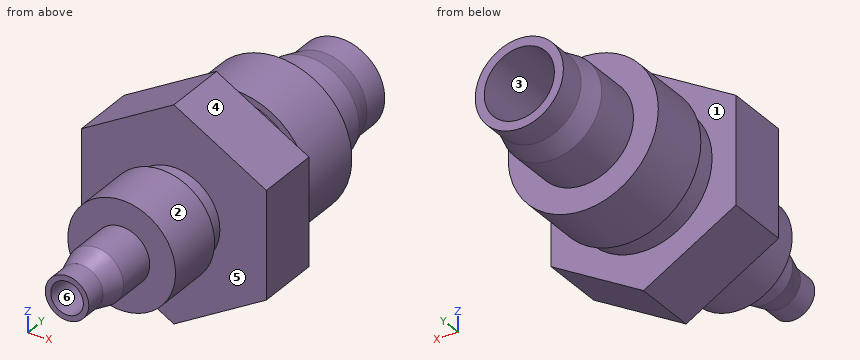
```python
from build123d import *

# Parameters (mm, degrees)
F1_DEPTH  = 3
F2_R      = 6.3
F3_DEPTH  = 2.5
F4_R      = 6.9
F5_DEPTH  = 6
F6_R      = 4.625
F7_DEPTH  = 4.5
F8_R      = 4.625
F9_DEPTH  = 2
F9_TAPER  = 16
F10_R     = 4.0515092285
F10_R_2   = 4
F11_DEPTH = 2.5
F12_R     = 3.225
F13_DEPTH = 20.5
F14_R     = 4.225
F15_DEPTH = 1.85
F16_R     = 4.95
F17_DEPTH = 5.5
F18_R     = 2.575
F19_DEPTH = 3.7
F20_R     = 2.575
F21_DEPTH = 2
F21_TAPER = 16
F22_R     = 2
F23_DEPTH = 2
F24_R     = 1.5
F25_DEPTH = 18.05
F26_R     = 3.225
F27_DEPTH = 3.5
F27_TAPER = 35


with BuildPart() as f1:
    # F0 (on Front) → F1 (new body, symmetric)
    with BuildSketch(Plane.XZ):
        Polygon((-8.5, -4.9074772881), (0, -9.8149545762), (8.5, -4.9074772881), (8.5, 4.9074772881), (0, 9.8149545762), (-8.5, 4.9074772881), align=None)
    extrude(amount=F1_DEPTH, both=True)

    # F2 (on face) → F3 (join)
    with BuildSketch(Plane(origin=(0, 3, 0), x_dir=(-1, 0, 0), z_dir=(0, 1, 0))):
        Circle(F2_R)
    extrude(amount=F3_DEPTH)

    # F4 (on face) → F5 (join)
    with BuildSketch(Plane(origin=(0, 5.5, 0), x_dir=(-1, 0, 0), z_dir=(0, 1, 0))):
        Circle(F4_R)
    extrude(amount=F5_DEPTH)

    # F6 (on face) → F7 (join)
    with BuildSketch(Plane(origin=(0, 11.5, 0), x_dir=(-1, 0, 0), z_dir=(0, 1, 0))):
        Circle(F6_R)
    extrude(amount=F7_DEPTH)

    # F8 (on face) → F9 (join)
    with BuildSketch(Plane(origin=(0, 16, 0), x_dir=(-1, 0, 0), z_dir=(0, 1, 0))):
        Circle(F8_R)
    extrude(amount=F9_DEPTH, taper=F9_TAPER)

    # F10 (on face) → F11 (join)
    with BuildSketch(Plane(origin=(0, 18, 0), x_dir=(-1, 0, 0), z_dir=(0, 1, 0))):
        Circle(F10_R)
        Circle(F10_R_2, mode=Mode.SUBTRACT)
        Circle(F10_R_2)
    extrude(amount=F11_DEPTH)

    # F12 (on face) → F13 (cut, through all)
    with BuildSketch(Plane(origin=(0, 20.5, 0), x_dir=(-1, 0, 0), z_dir=(0, 1, 0))):
        Circle(F12_R)
    extrude(amount=-F13_DEPTH, mode=Mode.SUBTRACT)

    # F14 (on face) → F15 (join)
    with BuildSketch(Plane.XZ.offset(3)):
        Circle(F14_R)
    extrude(amount=F15_DEPTH)

    # F16 (on face) → F17 (join)
    with BuildSketch(Plane.XZ.offset(4.85)):
        Circle(F16_R)
    extrude(amount=F17_DEPTH)

    # F18 (on face) → F19 (join)
    with BuildSketch(Plane.XZ.offset(10.35)):
        Circle(F18_R)
    extrude(amount=F19_DEPTH)

    # F20 (on face) → F21 (join)
    with BuildSketch(Plane.XZ.offset(14.05)):
        Circle(F20_R)
    extrude(amount=F21_DEPTH, taper=F21_TAPER)

    # F22 (on face) → F23 (join)
    with BuildSketch(Plane.XZ.offset(16.05)):
        Circle(F22_R)
    extrude(amount=F23_DEPTH)

    # F24 (on face) → F25 (cut, through all)
    with BuildSketch(Plane.XZ.offset(18.05)):
        Circle(F24_R)
    extrude(amount=-F25_DEPTH, mode=Mode.SUBTRACT)

    # F26 (on Front) → F27 (cut)
    with BuildSketch(Plane.XZ):
        Circle(F26_R)
    extrude(amount=F27_DEPTH, taper=F27_TAPER, mode=Mode.SUBTRACT)


solid = f1.part
```
Work out the finished part from the listing and answer in its coordinate system (mm). Face numbers are marked on the shaded views. A direction names the side the tool comes from. Round coordinates to 2 decimals unless told otherwise and drop trailing zeros. Write each loop counter-clockwise with the first axis right and the second up, starting at its lowest first coordinate (ties: lowest second). Pieces come first, ordered by that corner, then holes. Notation, with made-up numbers: (24.5, -16) - (72.5, -16) arc R9 cw to (72.5, -5) - close; hole circle Ø8 at (70.5, -13.75). An arc over 180 degrees is marked (long way). Return JSON: item names as keys, results as strings. Group by question number.
Q1. Find the intervals of material crossed by L1, parallel to Z at x = 0, y = -13.25 (3 decimals); L2, parallel to Y at x = 6, z = -3.25; L3, parallel to Z at x = 0, y = 14.75 (3 decimals), in increasing order.
Q2. The part is cut by section D-D on z = -8.25. Write down the section's boundary in (x, y), then the cut area to 3 significant figures.
Q3. For the marked faces 1, 2 and 3, determine the directions among +Z, -Z, +X, -X, +Y, -Y from which every point of the face is accessible in a straight line to the end or side of a thin tool.
Q4. Each of these flat-tipped pins is pushed along its axis until it touches: pin 1 Ø1 at (x, z) = (0, 7) entering from -Y; pin 2 Ø3 at (y, z) = (11.5, 4.5) entering from -X; pin 3 Ø10 at (x, y) = (-5.5, 11) entering from +Z. Where does it stop, or does it pass through?
Q5. The part is cut by section A-A on y = 2.5. Write down the section's boundary in (x, z) (3 decimals).
Q6. The mould has two halves that part along X. Classify the marked faces 4, 5 and 6: released by +X, released by -X, zero draft, split by the parting line, or undercut.
Q7. The part is cut by section C-C on y = 13. Write down the section's boundary in (x, z) (3 decimals), then the cut area to 3 significant figures.
Q8. The part is cut by section B-B on z = 5.5. Write down the section's boundary in (x, y), then the cut area to 3 significant figures.
Solved:
{
 "1": {"L1": "-2.575 to -1.5, 1.5 to 2.575", "L2": "-3 to 3, 5.5 to 11.5", "L3": "-4.625 to -3.225, 3.225 to 4.625"},
 "2": {"outline": "(-2.71, -3) - (2.71, -3) - (2.71, 3) - (-2.71, 3) - close", "area": "32.5 mm²"},
 "3": {"face 1": "none", "face 2": "-Y", "face 3": "+Y"},
 "4": {"pin 1": "y = -3", "pin 2": "x = -6.21", "pin 3": "z = 6.88"},
 "5": {"outline": "(-8.5, -4.907) - (0, -9.815) - (8.5, -4.907) - (8.5, 4.907) - (0, 9.815) - (-8.5, 4.907) - close; hole circle Ø6.45 at (0, 0)"},
 "6": {"face 4": "released by +X", "face 5": "zero draft", "face 6": "undercut"},
 "7": {"outline": "circle Ø9.25 at (0, 0); hole circle Ø6.45 at (0, 0)", "area": "34.5 mm²"},
 "8": {"outline": "(-7.47, -3) - (7.47, -3) - (7.47, 3) - (3.07, 3) - (3.07, 5.5) - (4.17, 5.5) - (4.17, 11.5) - (-4.17, 11.5) - (-4.17, 5.5) - (-3.07, 5.5) - (-3.07, 3) - (-7.47, 3) - close", "area": "155 mm²"}
}
